Geometry check sheet. Reference: drawing and pictorial views, mm from the part's lowest x, y, z. A direction names the side the tool comes from. Coordinates: 2 decimals unless noted, no trailing zeros. Loops run counter-clockwise (first coordinate to the right, second up) from the corner with the lowest first, then second, coordinate; pieces in that order, holes last. Notation, with made-up numbers: (-10, -28.75) - (27, -28.75) arc R14 ccw to (27, -14.75) - close; hole circle Ø5 at (-36.5, 11). An arc over 180 degrees is marked (long way). One line per item, written item: value.
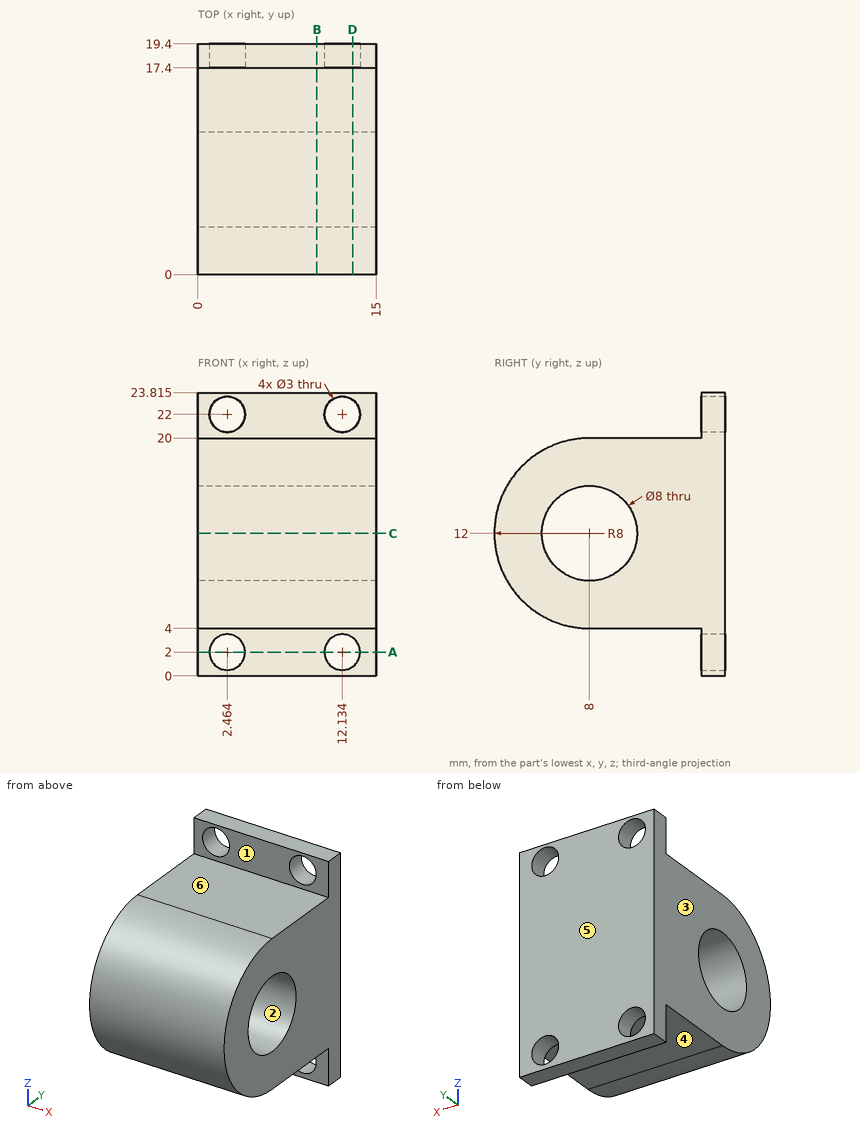
(1) Go/stop test with flat-tipped pins: pin 1 Ø1.9 at (x, z) = (6.5, 22.5) entering from -Y; pin 2 Ø8 at (x, y) = (11.5, 8) entering from -Z; pin 3 Ø6 at (y, z) = (5.5, 3.5) entering from +X; pin 4 Ø4 at (x, z) = (12.5, 16.5) entering from -Y. Record where each tip stops, or that it passes through.
Reply:
pin 1: y = 17.4
pin 2: z = 4
pin 3: x = 15
pin 4: y = 0.4
(2) Release check for a two-part mould opening along Y. For the marked faces 1, 2 and 3 record: pulls with the +Y half, pulls with the -Y half, needs draft (parallel to the pull), parting line crosses it, or undercut.
Reply:
face 1: pulls with the -Y half
face 2: undercut
face 3: needs draft
(3) Material ranges on probe 1 along X at (y, z) = (18.2, 2) (1 decimal); probe 2 along Z at (x, y) = (12, 18.75) (1 decimal); probe 3 along Y at (x, z) = (9.25, 12), recorded low to high. Write a range as from..to.
Reply:
probe 1: 0..1, 4..10.6, 13.6..15
probe 2: 0..0.5, 3.5..20.5, 23.5..23.8
probe 3: 0..4, 12..19.4
(4) Cross-section at D-D on x = 13. Record the cut outline in (y, z) (1 decimal).
Reply:
outline: (8, 4) - (17.4, 4) - (17.4, 3.2) - (19.4, 3.2) - (19.4, 20.8) - (17.4, 20.8) - (17.4, 20) - (8, 20) arc R8 ccw to start; (17.4, 0) - (19.4, 0) - (19.4, 0.8) - (17.4, 0.8) - close; (17.4, 23.2) - (19.4, 23.2) - (19.4, 23.8) - (17.4, 23.8) - close; hole circle Ø8 at (8, 12)
(5) Cross-section at C-C on z = 12. Record the cut outline in (x, y), and give its area (3 significant figures).
Reply:
outline: (0, 0) - (15, 0) - (15, 4) - (0, 4) - close; (0, 12) - (15, 12) - (15, 19.4) - (0, 19.4) - close
area: 171 mm2
(6) Access from +Z, -Z, +X, -X, +Y, -Y to the whole of each face (thin tool, end or side, straight path). Record for the marked faces 4, 5 and 6.
Reply:
face 4: -Z, +X, -X, -Y
face 5: +Z, -Z, +X, -X, +Y
face 6: +Z, +X, -X, -Y
(7) Cross-section at B-B on x = 10. Record the cut outline in (y, z) (1 decimal).
Reply:
outline: (8, 4) - (17.4, 4) - (17.4, 0) - (19.4, 0) - (19.4, 23.8) - (17.4, 23.8) - (17.4, 20) - (8, 20) arc R8 ccw to start; hole circle Ø8 at (8, 12)
(8) Cross-section at A-A on z = 2. Record the cut outline in (x, y) (1 decimal), and give its area (3 significant figures).
Reply:
outline: (0, 17.4) - (1, 17.4) - (1, 19.4) - (0, 19.4) - close; (4, 17.4) - (10.6, 17.4) - (10.6, 19.4) - (4, 19.4) - close; (13.6, 17.4) - (15, 17.4) - (15, 19.4) - (13.6, 19.4) - close
area: 18.0 mm2
